The model under review builds one solid part; all positions refer to its coordinate system, in mm. Face numbers are marked on the shaded views. A direction names the side the tool comes from. Round coordinates to 2 decimals unless told otherwise and drop trailing zeros. Loops run counter-clockwise (first coordinate to the right, second up) from the corner with the lowest first, then second, coordinate; pieces in that order, holes last. Notation, with made-up numbers: M 58.25,12 L 81.25,12 A33 cw 81.25,43 Z; hole C -9.5,49.25 d3. An arc over 180 degrees is marked long. Return JSON: item names as keys, results as strings. Group by question number.
Q1. Consider section B-B (y = 0). State the section outline as (x, z) points (3 decimals).
Q2. Consider section C-C (x = 0). State the section outline as (y, z) points (3 decimals), and give its area (3 significant figures).
Q3. Clearance check with flat-ended pins moving along their axes: pin 1 Ø8 at (x, y) = (-13, 208.5) entering from +Z; pin 2 Ø1.5 at (x, z) = (-43.5, 616) entering from +Y; pin 3 Ø6.5 at (x, z) = (-73, -52.5) entering from -Y. State where each tip first meets the part, or that it passes through.
Q4. Consider section A-A (z = 50.8). State the section outline as (x, y) points, and give its area (3 significant figures).
Q5. To check wall thickness, follow line 1 along X through (y, z) = (-14.5, 50.8); line 2 along Y through (x, z) = (0, 774) (3 decimals); line 3 along Z through (x, y) = (39, -18). State the ranges of each line that lie inside material, in increasing order.
Q6. Consider section D-D (z = 438.5). State the section outline as (x, y) points (3 decimals), and give its area (3 significant figures).
Q7. For the marked faces 1, 2, 3, 4 and 5, list the 3-axis set-ups (+Z, -Z, +X, -X, +Y, -Y) from which the entire face can be reached by the end or side of a thin tool; tool diameter is ignored.
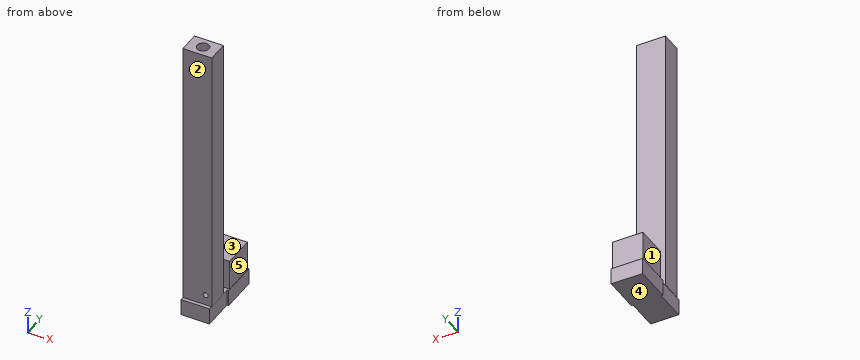
from build123d import *

# Parameters (mm, degrees)
SKETCH1_W               = 1310.386
SKETCH1_H               = 101.6
BOSS_EXTRUDE1_DEPTH     = 69.85
BOSS_EXTRUDE2_DEPTH     = 68.326
SKETCH3_W               = 79.430838384
SKETCH3_H               = 176.27
BOSS_EXTRUDE3_DEPTH     = 76.23
SKETCH4_W               = 146.04
SKETCH4_H               = 156.04
BOSS_EXTRUDE4_DEPTH     = 146.05
SKETCH5_R               = 28.575
CUT_EXTRUDE1_DEPTH      = 927.1
CUT_EXTRUDE2_DEPTH      = 10
CUT_EXTRUDE2_DEPTH_BACK = 1330.46311815
SKETCH6_R               = 12.7


with BuildPart() as part:
    # Sketch1 → Boss-Extrude1 (new, symmetric)
    with BuildSketch(Plane(origin=(0, 0, 0), x_dir=(0, 0, -1), z_dir=(1, 0, 0))):
        with Locations((-655.193, 0)):
            Rectangle(SKETCH1_W, SKETCH1_H)
    extrude(amount=BOSS_EXTRUDE1_DEPTH, both=True)

    # Sketch2 → Boss-Extrude2 (add, symmetric)
    with BuildSketch(Plane(origin=(0, 0, 0), x_dir=(0, 0, -1), z_dir=(1, 0, 0))):
        Polygon((0, 0), (0, -68.326), (79.430838384, -68.326), (79.430838384, 85.598), (0, 85.598), align=None)
    extrude(amount=BOSS_EXTRUDE2_DEPTH, both=True)

    # Sketch3 → Boss-Extrude3 (add, symmetric)
    with BuildSketch(Plane(origin=(0, 0, 0), x_dir=(0, 0, -1), z_dir=(1, 0, 0))):
        with Locations((39.715419192, 173.733)):
            Rectangle(SKETCH3_W, SKETCH3_H)
    extrude(amount=BOSS_EXTRUDE3_DEPTH, both=True)

    # Sketch4 → Boss-Extrude4 (add)
    with BuildSketch(Plane.XY):
        with Locations((1.79, 173.848)):
            Rectangle(SKETCH4_W, SKETCH4_H)
    extrude(amount=BOSS_EXTRUDE4_DEPTH)

    # Sketch5 → Cut-Extrude1 (cut)
    with BuildSketch(Plane.XY.offset(1310.386)):
        Circle(SKETCH5_R)
    extrude(amount=-CUT_EXTRUDE1_DEPTH, mode=Mode.SUBTRACT)

    # Sketch6 → Cut-Extrude2 (cut, two sides: drawn at the far end of the back side and taken through both)
    with BuildSketch(Plane(origin=(0, 50.8, 0), x_dir=(1, 0, 0), z_dir=(0, 1, 0)).offset(-CUT_EXTRUDE2_DEPTH_BACK)):
        with Locations(Location((39.81, -50.8, 0), (0, 0, 270))):
            Circle(SKETCH6_R)
    extrude(amount=CUT_EXTRUDE2_DEPTH + CUT_EXTRUDE2_DEPTH_BACK, mode=Mode.SUBTRACT)


solid = part.part
Values:
{
 "1": {"outline": "M -69.85,0 L -68.326,0 L -68.326,-79.431 L 68.326,-79.431 L 68.326,0 L 69.85,0 L 69.85,1310.386 L 28.575,1310.386 L 28.575,383.286 L -28.575,383.286 L -28.575,1310.386 L -69.85,1310.386 Z; hole C 39.81,50.8 d25.4"},
 "2": {"outline": "M -68.326,-79.431 L 261.868,-79.431 L 261.868,0 L 251.868,0 L 251.868,146.05 L 95.828,146.05 L 95.828,0 L 50.8,0 L 50.8,1310.386 L 28.575,1310.386 L 28.575,383.286 L -28.575,383.286 L -28.575,1310.386 L -50.8,1310.386 L -50.8,0 L -68.326,0 Z", "area": "129,000 mm2"},
 "3": {"pin 1": "stops at z = 146.05", "pin 2": "stops at y = 50.8", "pin 3": "stops at y = 85.6"},
 "4": {"outline": "M -71.23,95.83 L 74.81,95.83 L 74.81,251.87 L -71.23,251.87 Z; M -69.85,-50.8 L 27.11,-50.8 L 27.11,50.8 L -69.85,50.8 Z; M 52.51,-50.8 L 69.85,-50.8 L 69.85,50.8 L 52.51,50.8 Z", "area": "34,400 mm2"},
 "5": {"line 1": "x = -69.85 to 27.11, 52.51 to 69.85", "line 2": "y = -50.8 to -28.575, 28.575 to 50.8", "line 3": "z = -79.43 to 38.13, 63.47 to 1310.39"},
 "6": {"outline": "M -69.85,-50.8 L 69.85,-50.8 L 69.85,50.8 L -69.85,50.8 Z; hole C 0,0 d57.15", "area": "11,600 mm2"},
 "7": {"face 1": "+Z, -X, +Y, -Y", "face 2": "+Z, +X, -X, -Y", "face 3": "+Z, +X, -X, +Y", "face 4": "-Z, +X, -X, +Y, -Y", "face 5": "+Z, +X, +Y, -Y"}
}
